Source: CAD feature listing. Evaluate the final solid. Frame: model axes, mm. Face numbers are marked on the shaded views. Give positions to 0.01 mm unless a question says otherwise; leave off trailing zeros. Loops run counter-clockwise (first coordinate to the right, second up) from the corner with the lowest first, then second, coordinate; pieces in that order, holes last.
from build123d import *

# Parameters (mm, degrees)
ESQUISSE1_R             = 7.5
ESQUISSE1_R_2           = 4
BASE_EXTRUSION_DEPTH    = 4
CHANFREIN1_SIZE         = 0.8
ESQUISSE2_W             = 18
ESQUISSE2_H             = 18
ENL_V_MAT_EXTRU_1_DEPTH = 4


with BuildPart() as part:
    # Esquisse1 → Base-Extrusion (new body)
    with BuildSketch(Plane.XY):
        Circle(ESQUISSE1_R)
        Circle(ESQUISSE1_R_2, mode=Mode.SUBTRACT)
    extrude(amount=BASE_EXTRUSION_DEPTH)

    # Chanfrein1
    chanfrein1_edges = [part.edges().sort_by_distance(p)[0] for p in [
        (-7.5, 0, 0),
        (-7.5, 0, 4),
    ]]
    chamfer(chanfrein1_edges, length=CHANFREIN1_SIZE)

    # Esquisse2 → Enlèv. mat.-Extru.1 (cut)
    with BuildSketch(Plane.XY.offset(4)):
        Rectangle(ESQUISSE2_W, ESQUISSE2_H)
        Polygon((-7.5, 0), (-3.787466677, 6.43029634), (3.787466677, 6.43029634), (7.5, 0), (3.787466677, -6.43029634), (-3.787466677, -6.43029634), align=None, mode=Mode.SUBTRACT)
    extrude(amount=-ENL_V_MAT_EXTRU_1_DEPTH, mode=Mode.SUBTRACT)


solid = part.part
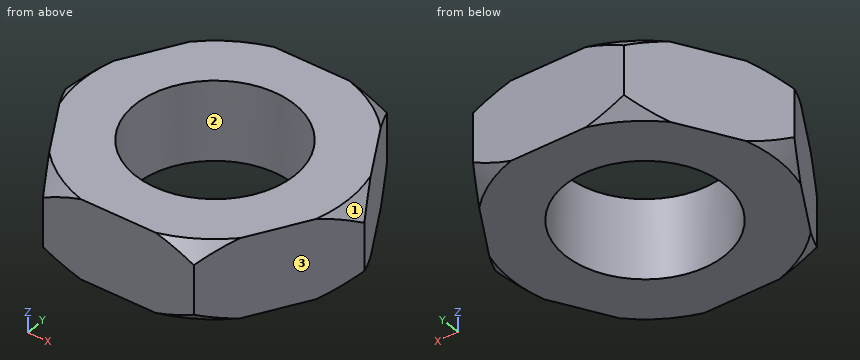
1) Cut plane A-A (x = 0). Return loops of the section in (y, z), and give its area (3 significant figures).
Checks:
outline: (-6.43, 0) - (-4, 0) - (-4, 4) - (-6.43, 4) - close; (4, 0) - (6.43, 0) - (6.43, 4) - (4, 4) - close
area: 19.4 mm2
2) Pull-direction query (Y, two-part tool) for the marked faces 1, 2 and 3; classes: released by +Y, released by -Y, zero draft, split by the parting line, or undercut.
Checks:
face 1: split by the parting line
face 2: undercut
face 3: released by -Y
3) Cut plane D-D (z = 3.5). Return loops of the section in (x, y), and give its area (3 significant figures).
Checks:
outline: (-7.18, -0.56) - (-4.07, -5.94) arc R7.2 ccw to (-3.24, -6.43) - (3.24, -6.43) arc R7.2 ccw to (4.07, -5.94) - (7.18, -0.56) arc R7.2 ccw to (7.18, 0.56) - (4.07, 5.94) arc R7.2 ccw to (3.24, 6.43) - (-3.24, 6.43) arc R7.2 ccw to (-4.07, 5.94) - (-7.18, 0.56) arc R7.2 ccw to start; hole circle Ø8 at (0, 0)
area: 94.1 mm2
4) Cut plane C-C (y = 3.75). Return loops of the section in (x, z).
Checks:
outline: (-5.33, 0) - (-1.39, 0) - (-1.39, 4) - (-5.33, 4) - close; (1.39, 0) - (5.33, 0) - (5.33, 4) - (1.39, 4) - close
5) Cut plane B-B (z = 1.75). Return loops of the section in (x, y), and give its area (3 significant figures).
Checks:
outline: (-7.5, 0) - (-3.79, -6.43) - (3.79, -6.43) - (7.5, 0) - (3.79, 6.43) - (-3.79, 6.43) - close; hole circle Ø8 at (0, 0)
area: 94.9 mm2
6) Contact query for flat-ended pins moving along their axis: P1, Ø2, axis at y = 2.5, z = 2.5, coming from the -X side; P2, Ø1.5, axis at x = -5, z = 0.5, coming from the -Y side. Output: stop coordinate, or through.
Checks:
P1: stops at x = -6.63
P2: stops at y = -5.63
7) Ray query, probe 1 along Y at (x, z) = (0, 1.1); probe 2 along Y at (x, z) = (1.5, 3.45); probe 3 along X at (y, z) = (1.25, 3.4). Return the intervals inside material, ascending.
Checks:
probe 1: y = -6.43 to -4, 4 to 6.43
probe 2: y = -6.43 to -3.71, 3.71 to 6.43
probe 3: x = -6.78 to -3.8, 3.8 to 6.78
